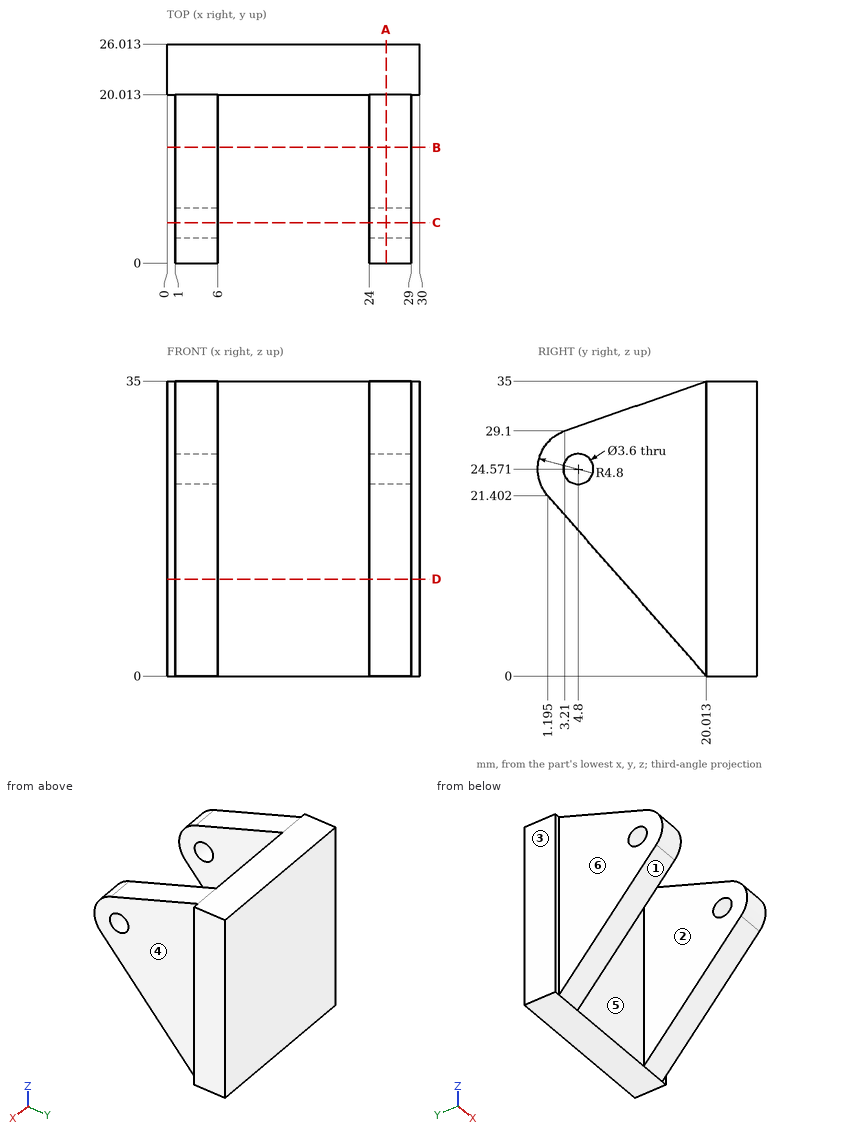
Drawing for the job (mm, zero at the part's lowest x, y, z). A direction names the side the tool comes from. Round coordinates to 2 decimals unless told otherwise and drop trailing zeros. Write each loop counter-clockwise with the first axis right and the second up, starting at its lowest first coordinate (ties: lowest second). Pieces come first, ordered by that corner, then holes.
Item 1: Band-saw the part on D-D on z = 11.5. Write the cut outline in (x, y).
Filled in:
outline: (0, 20.01) - (1, 20.01) - (1, 9.9) - (6, 9.9) - (6, 20.01) - (24, 20.01) - (24, 9.9) - (29, 9.9) - (29, 20.01) - (30, 20.01) - (30, 26.01) - (0, 26.01) - close
Item 2: Band-saw the part on B-B on y = 13.75. Write the cut outline in (x, z), then the cut area to 3 significant figures.
Filled in:
outline: (1, 7.12) - (6, 7.12) - (6, 32.8) - (1, 32.8) - close; (24, 7.12) - (29, 7.12) - (29, 32.8) - (24, 32.8) - close
area: 257 mm2
Item 3: Drop flat-ended pins along their axis: pin 1 Ø10 at (y, z) = (8.5, 11.5) entering from +X; pin 2 Ø1 at (x, z) = (18.5, 21.5) entering from -Y; pin 3 Ø1.5 at (x, z) = (25, 20.5) entering from -Y. Give the stop position or say it passes through.
Filled in:
pin 1: stops at x = 29
pin 2: stops at y = 20.01
pin 3: stops at y = 1.33
Item 4: Band-saw the part on C-C on y = 4.8. Write the cut outline in (x, z).
Filled in:
outline: (1, 17.3) - (6, 17.3) - (6, 22.77) - (1, 22.77) - close; (1, 26.37) - (6, 26.37) - (6, 29.66) - (1, 29.66) - close; (24, 17.3) - (29, 17.3) - (29, 22.77) - (24, 22.77) - close; (24, 26.37) - (29, 26.37) - (29, 29.66) - (24, 29.66) - close
Item 5: Tool access for the marked faces 4, 5 and 6: list every direction of +Z, -Z, +X, -X, +Y, -Y with a clear straight run to the whole face (end or side of a thin tool).
Filled in:
face 4: +Z, -Z, +X, -Y
face 5: +Z, -Z, -Y
face 6: +Z, -Z, -X, -Y
Item 6: Band-saw the part on A-A on x = 26. Write the cut outline in (y, z) (1 decimal), then the cut area to 3 significant figures.
Filled in:
outline: (1.2, 21.4) - (20, 0) - (26, 0) - (26, 35) - (20, 35) - (3.2, 29.1) arc R4.8 ccw to start; hole circle Ø3.6 at (4.8, 24.6)
area: 600 mm2
Item 7: Drill centre lines: L1, parallel to X at y = 7.5, z = 21.5; L2, parallel to Y at x = 17, z = 23.5; L3, parallel to Z at x = 26.8, y = 4.8 (1 decimal). Where is each one in solid material? Low to high.
Filled in:
L1: x = 1 to 6, 24 to 29
L2: y = 20.01 to 26.01
L3: z = 17.3 to 22.8, 26.4 to 29.7
Item 8: Mould opens along X. For the marked faces 1, 2 and 3 say: released by +X, released by -X, zero draft, split by the parting line, or undercut.
Filled in:
face 1: zero draft
face 2: undercut
face 3: released by -X
